Input: part model. Units: mm. Frame: model coordinates. A direction names the side the tool comes from. Round coordinates to 2 decimals unless told otherwise and drop trailing zeros. Write each loop counter-clockwise with the first axis right and the second up, starting at its lowest first coordinate (ties: lowest second). Pieces come first, ordered by that corner, then holes. Notation, with made-up numbers: (47.25, 48.25) -> (72.25, 48.25) arc R24 ccw to (72.25, 72.25) -> close; hole circle Ø2 at (67.5, -1.75). An arc over 180 degrees is marked (long way). Write item = value, one per line. Start each with the question number.
```python
from build123d import *

# Parameters (mm, degrees)
SKETCH1_R           = 24.875
BOSS_EXTRUDE1_DEPTH = 480
SKETCH4_R           = 47.5
BOSS_EXTRUDE2_DEPTH = 100
BOSS_EXTRUDE3_DEPTH = 200
CIRPATTERN1_COUNT   = 20


with BuildPart() as part:
    # Sketch1 → Boss-Extrude1 (new body)
    with BuildSketch(Plane.XY):
        Circle(SKETCH1_R)
    extrude(amount=BOSS_EXTRUDE1_DEPTH)

    # Sketch4 → Boss-Extrude2 (add, symmetric)
    with BuildSketch(Plane.XY.offset(240)):
        Circle(SKETCH4_R)
    extrude(amount=BOSS_EXTRUDE2_DEPTH, both=True)

    # Sketch5 → Boss-Extrude3 (add)
    with BuildSketch(Plane.XY.offset(340)):
        with BuildLine():
            ThreePointArc((7.5, 46.904157598), (0, 47.5), (-7.5, 46.904157598))
            Line((-7.5, 46.904157598), (-7.5, 37.5))
            Line((-7.5, 37.5), (7.5, 37.5))
            Line((7.5, 37.5), (7.5, 46.904157598))
        make_face()
        with BuildLine():
            Line((-7.5, 37.5), (-7.5, 46.904157598))
            ThreePointArc((-7.5, 46.904157598), (-30.822070015, -36.142080737), (47.5, 0))
            ThreePointArc((47.5, 0), (36.142080737, 30.822070015), (7.5, 46.904157598))
            Line((7.5, 46.904157598), (7.5, 37.5))
            Line((7.5, 37.5), (-7.5, 37.5))
        make_face()
        with BuildLine():
            Line((-3.5, 57.5), (-7.5, 52.5))
            Line((-7.5, 52.5), (-7.5, 46.904157598))
            ThreePointArc((-7.5, 46.904157598), (0, 47.5), (7.5, 46.904157598))
            Line((7.5, 46.904157598), (7.5, 52.5))
            Line((7.5, 52.5), (3.5, 57.5))
            Line((3.5, 57.5), (-3.5, 57.5))
        make_face()
    boss_extrude3 = extrude(amount=-BOSS_EXTRUDE3_DEPTH)

    # CirPattern1: Boss-Extrude3 ×20 about axis
    cirpattern1_axis = Axis((0, 0, 0), (0, 0, 1))
    for i in range(1, CIRPATTERN1_COUNT):
        add(boss_extrude3.rotate(cirpattern1_axis, i * 360 / CIRPATTERN1_COUNT))


solid = part.part
```
1. Line query: line 1 along Y through (x, z) = (36, 143); line 2 along Z through (x, y) = (8, -26.5); line 3 along X through (y, z) = (-11, 200). Output: solid intervals per line, ascending.
2. Pin query (flat end, axial travel): P1, Ø6, axis at y = -25.5, z = 392.5, coming from the +X side; P2, Ø1.5, axis at x = -1, y = 8, coming from the -Z side; P3, Ø5.5, axis at x = 50.5, z = 252, coming from the +Y side; P4, Ø3, axis at x = -9, z = 376, coming from the -Y side. Return the tip coordinate at first contact, or that it passes through.
3. Reachability of faces 1 (the flat face through (-1, 26, 140)), 2 (the flat face through (0, 0, 480)), 3 (the flat face through (-25, 9, 340)) from +Z, -Z, +X, -X, +Y, -Y: full face, straight path, thin tool, end or side. Return the list, or none.
4. Section A-A (z = 30). Output: boundary loops of the cut face in (x, y) (3 decimals).
Check sheet entries:
q1.line_1 = -44.92 to -36.79, -35.43 to 35.43, 36.79 to 44.92
q1.line_2 = 140 to 340
q1.line_3 = -53.5 to 53.5
q2.P1 = 10.61
q2.P2 = 0
q2.P3 = 32.1
q2.P4 = -23.72
q3.face_1 = -Z
q3.face_2 = +Z, +X, -X, +Y, -Y
q3.face_3 = +Z
q4.outline = circle Ø49.75 at (0, 0)
